from build123d import *

# Parameters (mm, degrees)
SKETCH328_W      = 15
SKETCH328_H      = 2
EXTRUDE197_DEPTH = 10
SKETCH327_W      = 9
SKETCH327_H      = 2
EXTRUDE196_DEPTH = 3
SKETCH326_W      = 31.550661
SKETCH326_H      = 34
EXTRUDE195_DEPTH = 2


with BuildPart() as extrude197:
    # Sketch328 → Extrude197 (new body)
    with BuildSketch(Plane(origin=(24.75, 6, 23), x_dir=(1, 0, 0), z_dir=(0, 0, 1))):
        with Locations((-69.5, 10)):
            Rectangle(SKETCH328_W, SKETCH328_H)
    extrude(amount=EXTRUDE197_DEPTH)


with BuildPart() as extrude197_1:
    # Extrude197 placement: moved
    add(extrude197.part.moved(Location((0, 0, -10))))


with BuildPart() as extrude196:
    # Sketch327 → Extrude196 (new body)
    with BuildSketch(Plane(origin=(-0.27, 0, 26), x_dir=(1, 0, 0), z_dir=(0, 0, 1))):
        with Locations((-44.5, 11)):
            Rectangle(SKETCH327_W, SKETCH327_H)
        with Locations((-44.5, -11)):
            Rectangle(SKETCH327_W, SKETCH327_H)
    extrude(amount=EXTRUDE196_DEPTH)


with BuildPart() as obj1:
    # Sketch326 → Extrude195 (new body)
    with BuildSketch(Plane.XY.offset(26)):
        with Locations((-39.224669, 0)):
            Rectangle(SKETCH326_W, SKETCH326_H)
    extrude(amount=EXTRUDE195_DEPTH)

    # Cut104: cut Extrude196
    add(extrude196.part, mode=Mode.SUBTRACT)


with BuildPart() as obj1_1:
    # Cut104 placement: moved
    add(obj1.part.moved(Location((0, 0, -10))))

    # Cut105: cut Extrude197
    add(extrude197_1.part, mode=Mode.SUBTRACT)


solid = obj1_1.part
Read the model definition and answer for the solid it produces. Units are mm, in the model's axes. A direction names the side the tool comes from. Give positions to 0.01 mm unless a question says otherwise; leave off trailing zeros. Loops run counter-clockwise (first coordinate to the right, second up) from the corner with the lowest first, then second, coordinate; pieces in that order, holes last. Notation, with made-up numbers: (55, -20) -> (72, -20) arc R25 cw to (72, 15) -> close; hole circle Ø8 at (0.5, 34.25). An arc over 180 degrees is marked (long way). Answer as CSV lines item,"result".
Item 1: For faces 1 (the face through (-54, 17, 17)), 2 (the face through (-45, 10, 17)), 3 (the face through (-37.25, 16, 17)), determine the directions among +Z, -Z, +X, -X, +Y, -Y from which every point of the face is accessible in a straight line to the end or side of a thin tool.
Returned:
face 1,"+Z, -Z, +X, -X, +Y"
face 2,"+Z, -Z"
face 3,"+Z, -Z, +Y"
Item 2: Determine the mould class of faces 4 (the face through (-39, 0, 18)), 5 (the face through (-45, 15, 17)), 6 (the face through (-40.27, -11, 17)) for opening direction Y: +Y half, -Y half, draft (parallel to the pull), parting line (faces both ways), or undercut.
Returned:
face 4,"draft"
face 5,"+Y half"
face 6,"undercut"
Item 3: Find section B-B on z = 17.3. Give the vertices of the cut face in (x, y), plus the area to 3 significant figures.
Returned:
outline,"(-55, -17) -> (-23.45, -17) -> (-23.45, 17) -> (-37.25, 17) -> (-37.25, 15) -> (-52.25, 15) -> (-52.25, 17) -> (-55, 17) -> close; hole (-49.27, -12) -> (-40.27, -12) -> (-40.27, -10) -> (-49.27, -10) -> close; hole (-49.27, 10) -> (-40.27, 10) -> (-40.27, 12) -> (-49.27, 12) -> close"
area,"1,010 mm²"
Item 4: This flat-tipped pin is pushed along its axis until it touches: pin 1 (0.6 mm diameter, centred on x = -46.5, z = 16.5, fed in from +Y). Where does it stop, or does it pass through?
Returned:
pin 1,"stops at y = 15"
Item 5: Consider line 1 (Y direction, x = -49, z = 16.95); line 2 (X direction, y = 16, z = 17.7); line 3 (Y direction, x = -40, z = 16.7). Determine where each line is inside the solid, lowest interval first. Write a range as [from, to].
Returned:
line 1,"y = [-17, -12], [-10, 10], [12, 15]"
line 2,"x = [-55, -52.25], [-37.25, -23.45]"
line 3,"y = [-17, 15]"
Item 6: Find section A-A on y = 11. Give the vertices of the cut face in (x, z).
Returned:
outline,"(-55, 16) -> (-49.27, 16) -> (-49.27, 18) -> (-55, 18) -> close; (-40.27, 16) -> (-23.45, 16) -> (-23.45, 18) -> (-40.27, 18) -> close"
Item 7: Find section D-D on x = -51. Give the vertices of the cut face in (y, z), plus the area to 3 significant figures.
Returned:
outline,"(-17, 16) -> (15, 16) -> (15, 18) -> (-17, 18) -> close"
area,"64.0 mm²"
Item 8: Find section C-C on x = -42.5. Give the vertices of the cut face in (y, z), plus the area to 3 significant figures.
Returned:
outline,"(-17, 16) -> (-12, 16) -> (-12, 18) -> (-17, 18) -> close; (-10, 16) -> (10, 16) -> (10, 18) -> (-10, 18) -> close; (12, 16) -> (15, 16) -> (15, 18) -> (12, 18) -> close"
area,"56.0 mm²"
